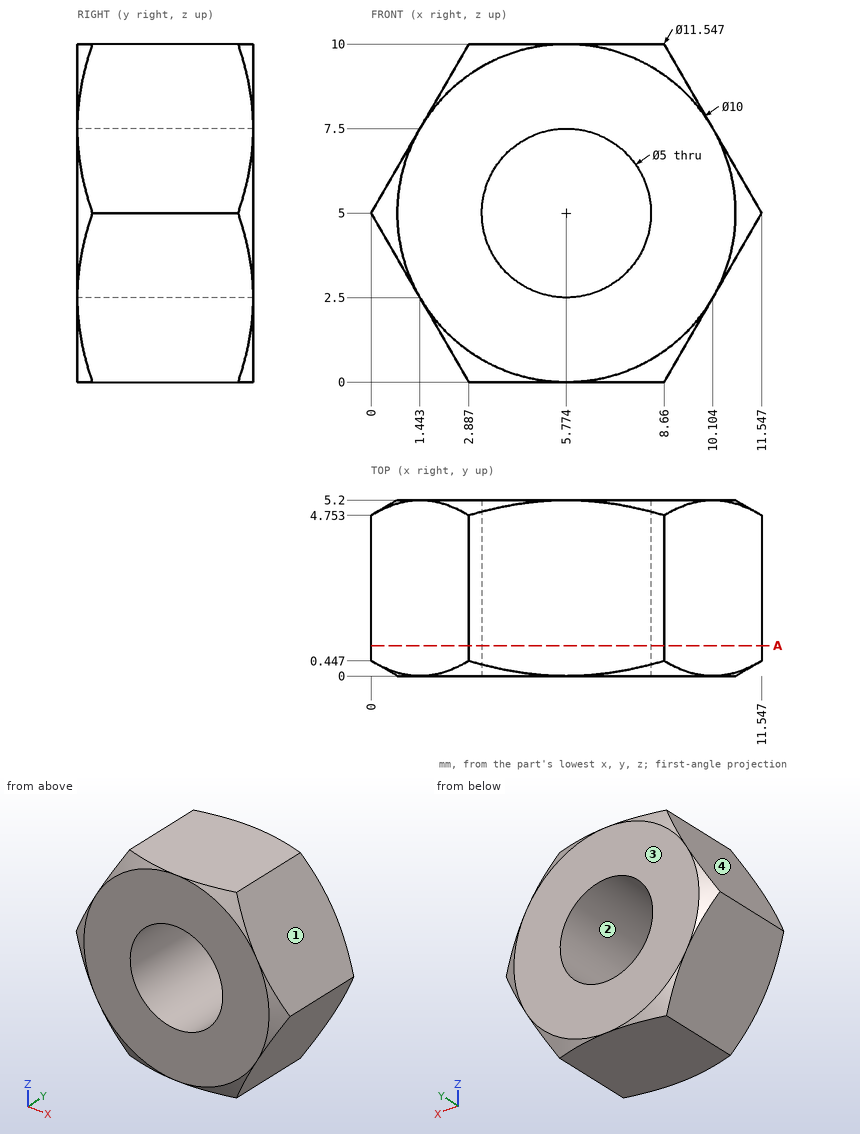
Study the drawing (mm; zero at the part's minimum x, y, z) and answer. Give positions to 0.01 mm unless a question says otherwise; leave off trailing zeros. Write each loop counter-clockwise with the first axis right and the second up, starting at its lowest first coordinate (ties: lowest second). Pieces come first, ordered by that corner, then holes.
(1) The mould has two halves that part along X. Classify the marked faces 1, 2, 3 and 4: pulls with the +X half, pulls with the -X half, needs draft (parallel to the pull), parting line crosses it, or undercut.
Final values:
face 1: pulls with the +X half
face 2: undercut
face 3: needs draft
face 4: pulls with the -X half
(2) A flat-ended cylindrical pin translates along its axis: pin 1 Ø3 at (x, z) = (5.77, 5) entering from -Y. Find the tip coordinate at first contact, or state that the pin passes through.
Final values:
pin 1: passes through
(3) The part is cut by section A-A on y = 0.9. Write down the section's boundary in (x, z).
Final values:
outline: (0, 5) - (2.89, 0) - (8.66, 0) - (11.55, 5) - (8.66, 10) - (2.89, 10) - close; hole circle Ø5 at (5.77, 5)
(4) Straight lines are drawn through the part: line 1 (Z direction, x = 5.75, y = 0.75); line 2 (Z direction, x = 7, y = 3.6); line 3 (X direction, y = 3.7, z = 3.5) (1 decimal). For each, find the intervals that lie inside material, in ascending order.
Final values:
line 1: z = 0 to 2.5, 7.5 to 10
line 2: z = 0 to 2.82, 7.18 to 10
line 3: x = 0.9 to 3.8, 7.8 to 10.7
